Autodesk Inventor part; units mm, degrees
ref_plane "YZ Plane" through (0, 0, 0) normal (1, 0, 0) x (0, 1, 0)
ref_plane "XZ Plane" through (0, 0, 0) normal (0, 1, 0) x (-1, 0, 0)
ref_plane "XY Plane" through (0, 0, 0) normal (0, 0, 1) x (1, 0, 0)
sketch "スケッチ1" plane through (0, 0, 0) normal (1, 0, 0) x (0, 1, 0)
  line L0 (0, 0) -> (-55.5, 0)
  line L1 (-55.5, 0) -> (-55.5, -54)
  line L2 (-55.5, -54) -> (0, -54)
  line L3 (0, -54) -> (0, 0)
  dimension "d0" = 55.5
  dimension "d1" = 54
extrude "押し出し1" add sketch "スケッチ1" along normal blind 5.5
sketch "スケッチ2" plane through (5.5, 0, 0) normal (1, 0, 0) x (0, 0, -1)
  line L0 (54, 0) -> (0, 0)
  line L1 (54, -55.5) -> (54, 0)
  line L2 (0, -55.5) -> (54, -55.5)
  line L3 (0, 0) -> (0, -55.5)
  point P0 (4.5, -4.5)
  point P1 (49.5, -4.5)
  point P2 (4.5, -51)
  point P3 (49.5, -51)
  dimension "d4" = 4.5
  dimension "d5" = 4.5
  dimension "d6" = 4.5
  dimension "d7" = 4.5
  dimension "d8" = 4.5
  dimension "d9" = 4.5
  dimension "d10" = 4.5
  dimension "d11" = 4.5
hole "穴1" at (5.5, -4.5, -4.5) at (5.5, -4.5, -49.5) at (5.5, -51, -4.5) at (5.5, -51, -49.5) direction (-1, 0, 0) diameter 3 end through all
sketch "スケッチ3" plane through (5.5, 0, 0) normal (1, 0, 0) x (0, 0, -1)
  line L0 (54, 0) -> (0, 0)
  line L1 (0, -55.5) -> (54, -55.5)
  circle A0 centre (4.5, -51) radius 1.5
  circle A1 centre (4.5, -4.5) radius 1.5
  point P0 (13, -4.5)
  point P1 (13, -51)
  dimension "d19" = 4.5
  dimension "d20" = 4.5
  dimension "d21" = 8.5
  dimension "d22" = 8.5
hole "穴2" at (5.5, -4.5, -13) at (5.5, -51, -13) direction (-1, 0, 0) diameter 4 end through all
sketch "スケッチ4" plane through (0, 0, 0) normal (-1, 0, 0) x (0, 0, 1)
  line L0 (-30, -14.25) -> (-30, -29.75)
  line L1 (-30, -14.25) -> (-14.5, -14.25) construction
  line L2 (-30, -29.75) -> (-16.5766, -37.5)
  line L3 (-30, -29.75) -> (-43.4234, -37.5)
  line L4 (-30, -29.75) -> (-14.5, -29.75) construction
  circle A0 centre (-43.4234, -37.5) radius 1.5
  circle A1 centre (-16.5766, -37.5) radius 1.5
  circle A2 centre (-30, -14.25) radius 1.5
  circle A3 centre (-37, -29.75) radius 6
  line L5 (0, -55.5) -> (-54, -55.5)
  line L6 (-54, 0) -> (0, 0)
  line L7 (-54, -55.5) -> (-54, 0)
  dimension "d30" = 15.5
  dimension "d31" = 90
  dimension "d32" = 15.5
  dimension "d33" = 120
  dimension "d34" = 15.5
  dimension "d35" = 150
  dimension "d36" = 3
  dimension "d37" = 3
  dimension "d38" = 3
  dimension "d42" = 12
  dimension "d43" = 7
  dimension "d44" = 0
  dimension "d47" = 25.75
  dimension "d48" = 55.5
  dimension "d49" = 24
extrude "押し出し3" cut sketch "スケッチ4" against normal blind 10
sketch "スケッチ5" plane through (0, 0, 0) normal (0, 1, 0) x (1, 0, 0)
  line L0 (0, 0) -> (5.5, 0)
  line L1 (5.5, 0) -> (5.5, 54)
  line L2 (0, 0) -> (5.5, 0)
  line L3 (5.5, 0) -> (5.5, 54)
  line L4 (5.5, 54) -> (0, 54)
  line L5 (0, 54) -> (0, 0)
extrude "押し出し4" add sketch "スケッチ5" along normal blind 25
fillet "フィレット2" radius 8 2 edges at (2.75, 25, -54) (2.75, 25, 0)
fillet "フィレット3" radius 4.5 2 edges at (2.75, -55.5, -54) (2.75, -55.5, 0)
sketch "スケッチ6" plane through (0, 0, 0) normal (-1, 0, 0) x (0, 0, 1)
  line L0 (-46, 25) -> (-8, 25)
  circle A0 centre (-37, -29.75) radius 6
  line L1 (-54, -51) -> (-54, 17)
  point P0 (0, 0)
  point P1 (-37, 18)
  dimension "d55" = 7
  dimension "d56" = 17
  dimension "d57" = 17
hole "穴3" at (0, 18, -37) direction (1, 0, 0) diameter 8 end through all
sketch "スケッチ7" plane through (0, 0, 0) normal (-1, 0, 0) x (0, 0, 1)
  line L0 (-46, 25) -> (-8, 25)
  line L1 (0, -51) -> (0, 17)
  point P0 (0, 0)
  point P1 (-10, 15)
  point P2 (-15, 15)
  point P3 (-20, 15)
  point P4 (-25, 15)
  point P5 (-10, 10)
  point P6 (-15, 10)
  point P7 (-20, 10)
  point P8 (-25, 10)
  point P9 (-10, 5)
  point P10 (-15, 5)
  point P11 (-20, 5)
  point P12 (-25, 5)
  point P13 (-10, 0)
  point P14 (-15, 0)
  point P15 (-20, 0)
  point P16 (-25, 0)
  point P17 (-10, 20)
  point P18 (-15, 15)
  point P19 (-15, 20)
  point P20 (-20, 15)
  point P21 (-20, 20)
  point P22 (-25, 15)
  point P23 (-25, 20)
  point P24 (-30, 15)
  point P25 (-30, 20)
  point P26 (-5, 15)
  point P27 (-10, 10)
  point P28 (-5, 10)
  point P29 (-10, 5)
  point P30 (-5, 5)
  point P31 (-10, 0)
  point P32 (-5, 0)
  point P33 (-30, 10)
  point P34 (-35, 10)
  point P35 (-40, 10)
  point P36 (-45, 10)
  point P37 (-25, 5)
  point P38 (-30, 5)
  point P39 (-35, 5)
  point P40 (-40, 5)
  point P41 (-45, 5)
  point P42 (-25, 0)
  point P43 (-30, 0)
  point P44 (-35, 0)
  point P45 (-40, 0)
  point P46 (-45, 0)
  dimension "d65" = 10
  dimension "d66" = 10
  dimension "d69" = 5
  dimension "d72" = 5
  dimension "d77" = 5
  dimension "d80" = 5
  dimension "d85" = 5
  dimension "d88" = 5
  dimension "d93" = 5
  dimension "d96" = 5
hole "穴4" at (0, 15, -10) at (0, 15, -15) at (0, 15, -20) at (0, 15, -25) at (0, 10, -10) at (0, 10, -15) at (0, 10, -20) at (0, 10, -25) at (0, 5, -10) at (0, 5, -15) at (0, 5, -20) at (0, 5, -25) at (0, 0, -10) at (0, 0, -15) at (0, 0, -20) at (0, 0, -25) at (0, 20, -10) at (0, 20, -15) at (0, 20, -20) at (0, 20, -25) at (0, 15, -30) at (0, 20, -30) at (0, 15, -5) at (0, 10, -5) at (0, 5, -5) at (0, 0, -5) at (0, 10, -30) at (0, 10, -35) at (0, 10, -40) at (0, 10, -45) at (0, 5, -30) at (0, 5, -35) at (0, 5, -40) at (0, 5, -45) at (0, 0, -30) at (0, 0, -35) at (0, 0, -40) at (0, 0, -45) direction (1, 0, 0) diameter 4 end through all
properties part number "ハンド_モータパネル" material "木材 (カエデ材)"
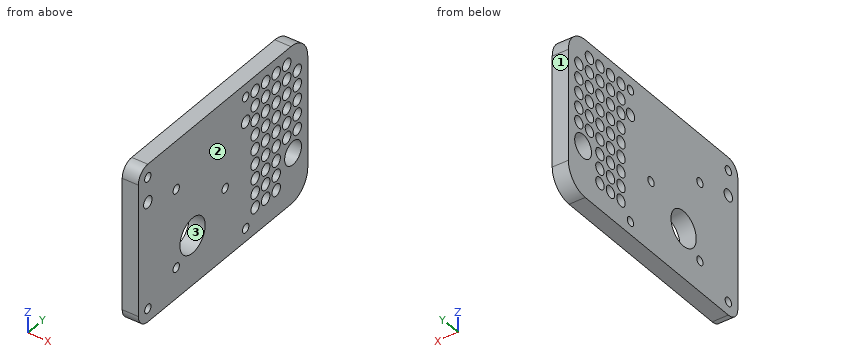
Check sheet for the modelled part. Datum: model origin and axes. Units: mm. Face numbers are marked on the shaded views. Coordinates: 2 decimals unless noted, no trailing zeros. Loops run counter-clockwise (first coordinate to the right, second up) from the corner with the lowest first, then second, coordinate; pieces in that order, holes last. Notation, with made-up numbers: (41, 7.5) -> (86, 7.5) arc R26 ccw to (86, 34.5) -> close; hole circle Ø8 at (-30.75, 37.25). An arc over 180 degrees is marked (long way). Write item = value, one per line. Start each with the question number.
1. Section check A-A on z = -20. Record the cut outline in (x, y).
2. Section check C-C on z = -14. Give the number of separate pieces and of enclosed holes in the cut face, then the cut area to 3 significant figures.
3. Material ranges on line 1 (Z direction, x = 2.7, y = -37.5); line 2 (Y direction, x = 2.4, z = -6.5); line 3 (Y direction, x = 4.7, z = -33.5), recorded low to high.
4. Draft check along Y on the marked faces 1, 2 and 3. Enter one of: released by +Y, released by -Y, zero draft, split by the parting line, or undercut.
5. Section check B-B on y = -29.75. Record the cut outline in (x, z).
Responses:
q1.outline = (0, -55.5) -> (5.5, -55.5) -> (5.5, -2) -> (0, -2) -> close; (0, 2) -> (5.5, 2) -> (5.5, 3) -> (0, 3) -> close; (0, 7) -> (5.5, 7) -> (5.5, 8) -> (0, 8) -> close; (0, 12) -> (5.5, 12) -> (5.5, 13) -> (0, 13) -> close; (0, 17) -> (5.5, 17) -> (5.5, 18) -> (0, 18) -> close; (0, 22) -> (5.5, 22) -> (5.5, 25) -> (0, 25) -> close
q2.separate_pieces = 8
q2.enclosed_holes = 0
q2.area = 309 mm2
q3.line_1 = -54 to -44.92, -41.92 to -18.08, -15.08 to 0
q3.line_2 = -55.5 to -1.32, 1.32 to 3.68, 6.32 to 8.68, 11.32 to 13.68, 16.32 to 24.86
q3.line_3 = -55.5 to -34.62, -24.88 to -1.32, 1.32 to 3.68, 6.32 to 8.68, 11.32 to 16.06, 19.94 to 25
q4.face_1 = released by +Y
q4.face_2 = zero draft
q4.face_3 = undercut
q5.outline = (0, -54) -> (5.5, -54) -> (5.5, -43) -> (0, -43) -> close; (0, -31) -> (5.5, -31) -> (5.5, 0) -> (0, 0) -> close
